Verification items for the finished model (mm, model axes). Coordinates: 2 decimals unless noted, no trailing zeros. Loops run counter-clockwise (first coordinate to the right, second up) from the corner with the lowest first, then second, coordinate; pieces in that order, holes last.
Q1. Mould release check, pull along X, two halves, no side actions. Record for faces 1 (the face through (-2, 0, -1)), 2 (the face through (148, 5, 1)), 3 (the face through (-113.784, 4.93, 71.812)), 4 (the face through (-148, 5, 1)): +X half, -X half, draft (parallel to the pull), parting line (faces both ways), or undercut.
Q2. Sectioned sample at B-B (z = -74.5). Enter the section's corners in (x, y).
Q3. Go/stop test with a flat-tipped pin: P1, Ø9, axis at x = 118, z = 74.5, coming from the +Y side. Record where the tip stops, or that it passes through.
Q4. Sectioned sample at A-A (x = 0). Enter the section's corners in (y, z), then the cut area to 3 significant figures.
Q5. Material ranges on probe 1 along X at (y, z) = (4, 74.5); probe 2 along X at (y, z) = (6, -74.5); probe 3 along Z at (x, y) = (-121, 5.75), recorded low to high.
```python
from build123d import *

# Parameters (mm, degrees)
SKETCH1_W          = 296
SKETCH1_H          = 209
EXTRUDE1_DEPTH     = 10
CUT_EXTRUDE1_REACH = 183.45
SKETCH2_R          = 5


with BuildPart() as part:
    # Sketch1 → Extrude1 (new body)
    with BuildSketch(Plane(origin=(0, 0, 0), x_dir=(1, 0, 0), z_dir=(0, 1, 0))):
        Rectangle(SKETCH1_W, SKETCH1_H)
    extrude(amount=EXTRUDE1_DEPTH)

    # Sketch2 → Cut-Extrude1 (cut, up to next)
    with BuildSketch(Plane.XZ, mode=Mode.PRIVATE) as cut_extrude1_sk1:
        with Locations(Location((-118, 74.5, 0), (0, 0, 270))):
            Circle(SKETCH2_R)
    cut_extrude1_tool1 = extrude(cut_extrude1_sk1.sketch, amount=-CUT_EXTRUDE1_REACH, mode=Mode.PRIVATE) & part.part
    # Sketch2 → Cut-Extrude1 (cut, up to next)
    with BuildSketch(Plane.XZ, mode=Mode.PRIVATE) as cut_extrude1_sk2:
        with Locations(Location((118, 74.5, 0), (0, 0, 270))):
            Circle(SKETCH2_R)
    cut_extrude1_tool2 = extrude(cut_extrude1_sk2.sketch, amount=-CUT_EXTRUDE1_REACH, mode=Mode.PRIVATE) & part.part
    # Sketch2 → Cut-Extrude1 (cut, up to next)
    with BuildSketch(Plane.XZ, mode=Mode.PRIVATE) as cut_extrude1_sk3:
        with Locations(Location((0, -74.5, 0), (0, 0, 270))):
            Circle(SKETCH2_R)
    cut_extrude1_tool3 = extrude(cut_extrude1_sk3.sketch, amount=-CUT_EXTRUDE1_REACH, mode=Mode.PRIVATE) & part.part
    add(cut_extrude1_tool1.solids().sort_by_distance((-118, 0, 74.5))[0], mode=Mode.SUBTRACT)
    add(cut_extrude1_tool2.solids().sort_by_distance((118, 0, 74.5))[0], mode=Mode.SUBTRACT)
    add(cut_extrude1_tool3.solids().sort_by_distance((0, 0, -74.5))[0], mode=Mode.SUBTRACT)


solid = part.part
```
Geometry check:
1. face 1: draft
1. face 2: +X half
1. face 3: undercut
1. face 4: -X half
2. outline: (-148, 0) - (-5, 0) - (-5, 10) - (-148, 10) - close; (5, 0) - (148, 0) - (148, 10) - (5, 10) - close
3. P1: passes through
4. outline: (0, -104.5) - (10, -104.5) - (10, -79.5) - (0, -79.5) - close; (0, -69.5) - (10, -69.5) - (10, 104.5) - (0, 104.5) - close
4. area: 1,990 mm2
5. probe 1: x = -148 to -123, -113 to 113, 123 to 148
5. probe 2: x = -148 to -5, 5 to 148
5. probe 3: z = -104.5 to 70.5, 78.5 to 104.5
